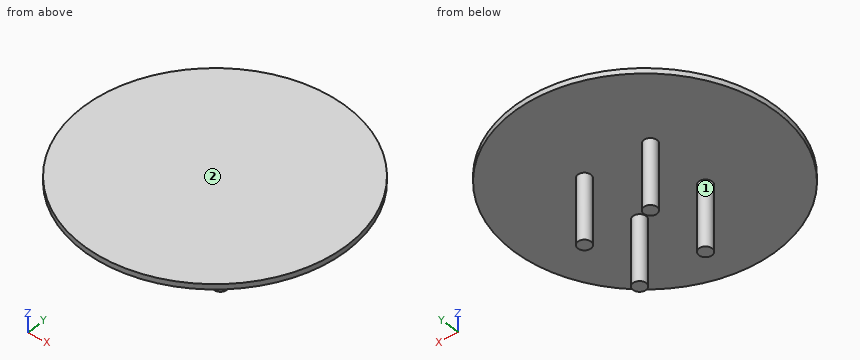
from build123d import *

# Parameters (mm, degrees)
F0_R     = 2.5
F1_DEPTH = 25
F2_R     = 50
F2_R_2   = 2.5
F3_DEPTH = 25
F5_R     = 50
F5_R_2   = 2.5
F6_DEPTH = 2


with BuildPart() as f1:
    # F0 (on Top) → F1 (new body)
    with BuildSketch(Plane.XY):
        with Locations((12.5, 12.5)):
            Circle(F0_R)
        with Locations((-12.5, -12.5)):
            Circle(F0_R)
        with Locations((12.5, -12.5)):
            Circle(F0_R)
        with Locations((-12.5, 12.5)):
            Circle(F0_R)
    extrude(amount=F1_DEPTH)

    # F5 (on face) → F6 (join)
    with BuildSketch(Plane.XY.offset(25)):
        Circle(F5_R)
        with Locations((12.5, 12.5)):
            Circle(F5_R_2, mode=Mode.SUBTRACT)
        with Locations((12.5, 12.5)):
            Circle(F5_R_2)
    extrude(amount=F6_DEPTH)


with BuildPart() as f3:
    # F2 (on face) → F3 (new body)
    with BuildSketch(Plane.XY.offset(25)):
        Circle(F2_R)
        with Locations((12.5, 12.5)):
            Circle(F2_R_2, mode=Mode.SUBTRACT)
    extrude(amount=F3_DEPTH)


solid = f1.part
The listing builds one solid part. Answer for the finished solid, in the listing's coordinates (mm). Face numbers are marked on the shaded views. Give positions to 0.01 mm unless a question says otherwise; leave off trailing zeros. Write each loop counter-clockwise with the first axis right and the second up, starting at its lowest first coordinate (ties: lowest second). Pieces come first, ordered by that corner, then holes.
1) Find the intervals of material crossed by L1, parallel to Z at x = 13, y = -3.5; L2, parallel to X at y = -12, z = 14, in increasing order.
2) Section D-D (x = 0) is taken. Write down the section's boundary in (y, z).
3) Section C-C (z = 9.5) is taken. Write down the section's boundary in (x, y), and give its area (3 significant figures).
4) Section A-A (y = 12.5) is taken. Write down the section's boundary in (x, z).
5) For a pull along X with two mould halves and no side action, classify the marked faces 1 and 2 as pulls with the +X half, pulls with the -X half, needs draft (parallel to the pull), parting line crosses it, or undercut.
6) Given P1, Ø6, axis at x = -15, z = 12, coming from the +Y side; P2, Ø8, axis at x = 1, z = 21.5, coming from the -Y side; P3, Ø1, axis at x = -23, y = -16, coming from the -Z side, each flat-ended and moving along its own axis, determine where each tip first touches the part or whether it passes through.
Response:
1. L1: z = 25 to 27
1. L2: x = -14.95 to -10.05, 10.05 to 14.95
2. outline: (-50, 25) - (50, 25) - (50, 27) - (-50, 27) - close
3. outline: circle Ø5 at (-12.5, -12.5); circle Ø5 at (-12.5, 12.5); circle Ø5 at (12.5, -12.5); circle Ø5 at (12.5, 12.5)
3. area: 78.5 mm2
4. outline: (-48.41, 25) - (-15, 25) - (-15, 0) - (-10, 0) - (-10, 25) - (10, 25) - (10, 0) - (15, 0) - (15, 25) - (48.41, 25) - (48.41, 27) - (-48.41, 27) - close
5. face 1: undercut
5. face 2: needs draft
6. P1: stops at y = 15
6. P2: stops at y = -50
6. P3: stops at z = 25
